Input: part model. Units: mm. Frame: model coordinates. A direction names the side the tool comes from. Round coordinates to 2 decimals unless told otherwise and drop trailing zeros. Loops run counter-clockwise (first coordinate to the right, second up) from the corner with the lowest first, then second, coordinate; pieces in that order, holes last.
1) Section D-D, the plane z = 13.5. Return loops of the section in (x, y), and give its area (3 significant figures).
2) Section A-A, the plane y = 0. Return loops of the section in (x, z).
3) Access query for faces 1 (the face through (-7.5, -3, 7)), 2 (the face through (0, -9, 18)). Directions: +Z, -Z, +X, -X, +Y, -Y. A direction counts if a zero-diameter tool reaches every point of the face in a straight line with its end or side. Return the directions, or none.
4) Draft query along X for faces 3 (the face through (10.5, -3, 7)), 4 (the face through (-2, 3, 3)), 5 (the face through (2, -3, 0)), 6 (the face through (7.5, -3, 7)). Return one class per face: pulls with the +X half, pulls with the -X half, needs draft (parallel to the pull), parting line crosses it, or undercut.
5) Section B-B, the plane z = 10.5. Return loops of the section in (x, y), and give its area (3 significant figures).
6) Ray query, line 1 along Y through (x, z) = (0, 0.7); line 2 along Z through (x, y) = (0, -8.2); line 3 along X through (y, z) = (-0.25, 3.75). Return the intervals inside material, ascending.
7) Section C-C, the plane x = -2.75. Return loops of the section in (y, z).
8) First-contact query: pin 1 (5 mm diameter, centred on x = 2.5, y = -2.5, fed in from +Z); pin 2 (7.5 mm diameter, centred on x = -2, z = 8.5, fed in from +Y). Flat tips, straight axial feed; report the tip coordinate or a pass-through.
from build123d import *

# Parameters (mm, degrees)
SKETCH1_W           = 15
SKETCH1_H           = 15
SKETCH1_R           = 3.302
BOSS_EXTRUDE1_DEPTH = 3
SKETCH2_W           = 15
SKETCH2_H           = 18
SKETCH2_R           = 1.65
BOSS_EXTRUDE2_DEPTH = 3
BOSS_EXTRUDE3_DEPTH = 3


with BuildPart() as part:
    # Sketch1 → Boss-Extrude1 (new body)
    with BuildSketch(Plane.XY):
        Rectangle(SKETCH1_W, SKETCH1_H)
        Circle(SKETCH1_R, mode=Mode.SUBTRACT)
    extrude(amount=BOSS_EXTRUDE1_DEPTH)

    # Sketch2 → Boss-Extrude2 (add)
    with BuildSketch(Plane.XZ.offset(7.5)):
        with Locations((0, 9)):
            Rectangle(SKETCH2_W, SKETCH2_H)
        with Locations((0, 10.5)):
            Circle(SKETCH2_R, mode=Mode.SUBTRACT)
    extrude(amount=BOSS_EXTRUDE2_DEPTH)

    # Sketch3 → Boss-Extrude3 (add)
    with BuildSketch(Plane(origin=(7.5, 0, 0), x_dir=(0, 0, -1), z_dir=(1, 0, 0))):
        Polygon((-18, -10.5), (-18, -7.5), (-3, 7.5), (0, 7.5), (0, -10.5), align=None)
    boss_extrude3 = extrude(amount=BOSS_EXTRUDE3_DEPTH)

    # Mirror1: Boss-Extrude3 across plane
    add(boss_extrude3.mirror(Plane(origin=(0, 0, 0), x_dir=(0, 0, 1), z_dir=(1, 0, 0))))


solid = part.part
Final values:
1. outline: (-10.5, -10.5) - (10.5, -10.5) - (10.5, -3) - (7.5, -3) - (7.5, -7.5) - (-7.5, -7.5) - (-7.5, -3) - (-10.5, -3) - close
1. area: 90.0 mm2
2. outline: (-10.5, 0) - (-3.3, 0) - (-3.3, 3) - (-7.5, 3) - (-7.5, 10.5) - (-10.5, 10.5) - close; (3.3, 0) - (10.5, 0) - (10.5, 10.5) - (7.5, 10.5) - (7.5, 3) - (3.3, 3) - close
3. face 1: +Z, +Y
3. face 2: +Z, +X, -X, +Y, -Y
4. face 3: pulls with the +X half
4. face 4: undercut
4. face 5: needs draft
4. face 6: undercut
5. outline: (-10.5, -10.5) - (-1.65, -10.5) - (-1.65, -7.5) - (-7.5, -7.5) - (-7.5, 0) - (-10.5, 0) - close; (1.65, -10.5) - (10.5, -10.5) - (10.5, 0) - (7.5, 0) - (7.5, -7.5) - (1.65, -7.5) - close
5. area: 98.1 mm2
6. line 1: y = -10.5 to -3.3, 3.3 to 7.5
6. line 2: z = 0 to 8.85, 12.15 to 18
6. line 3: x = -10.5 to -7.5, 7.5 to 10.5
7. outline: (-10.5, 0) - (-1.83, 0) - (-1.83, 3) - (-7.5, 3) - (-7.5, 18) - (-10.5, 18) - close; (1.83, 0) - (7.5, 0) - (7.5, 3) - (1.83, 3) - close
8. pin 1: stops at z = 3
8. pin 2: stops at y = -7.5
